CAD build for the part. Positions are in the model's coordinates, mm. Give positions to 0.01 mm unless a question says otherwise; leave off trailing zeros. Write each loop counter-clockwise with the first axis right and the second up, starting at its lowest first coordinate (ties: lowest second). Pieces come first, ordered by that corner, then holes. Notation, with made-up numbers: (71, -38) - (77, -38) arc R13 cw to (77, -20) - close; hole circle Ø4 at (-21, 33.5). An arc over 180 degrees is marked (long way). Answer as a JSON object with one key per item and string values.
from build123d import *

# Parameters (mm, degrees)
SKETCH2_R           = 5.08
BOSS_EXTRUDE1_DEPTH = 6.35
FILLET1_R           = 6.35
FILLET2_R           = 6.35


with BuildPart() as part:
    # Sketch2 → Boss-Extrude1 (new body)
    with BuildSketch(Plane(origin=(0, 0, 0), x_dir=(1, 0, 0), z_dir=(0, 1, 0))):
        Polygon((-152.4, 152.4), (-152.4, -152.4), (152.4, -152.4), (152.4, 142.494), (152.4, 152.4), (142.494, 152.4), align=None)
        with Locations((-139.7, -139.7)):
            Circle(SKETCH2_R, mode=Mode.SUBTRACT)
        with Locations((-56.896, -76.2)):
            Circle(SKETCH2_R, mode=Mode.SUBTRACT)
        with Locations((139.7, -139.7)):
            Circle(SKETCH2_R, mode=Mode.SUBTRACT)
        with Locations((56.896, -76.2)):
            Circle(SKETCH2_R, mode=Mode.SUBTRACT)
        with Locations((-139.7, 139.7)):
            Circle(SKETCH2_R, mode=Mode.SUBTRACT)
        with Locations((-31.496, 88.9)):
            Circle(SKETCH2_R, mode=Mode.SUBTRACT)
        with Locations((31.496, 88.9)):
            Circle(SKETCH2_R, mode=Mode.SUBTRACT)
        with Locations((139.7, 139.7)):
            Circle(SKETCH2_R, mode=Mode.SUBTRACT)
    extrude(amount=BOSS_EXTRUDE1_DEPTH)

    # Fillet1
    fillet1_edges = [part.edges().sort_by_distance(p)[0] for p in [
        (-152.4, 3.175, 152.4),
    ]]
    fillet(fillet1_edges, radius=FILLET1_R)

    # Fillet2
    fillet2_edges = [part.edges().sort_by_distance(p)[0] for p in [
        (-152.4, 3.175, -152.4),
        (152.4, 3.175, -152.4),
        (152.4, 3.175, 152.4),
    ]]
    fillet(fillet2_edges, radius=FILLET2_R)


solid = part.part
(1) Flat gauge pins, fed straight in: P1, Ø16.5, axis at x = 139.7, z = 139.7, coming from the -Y side; P2, Ø6, axis at x = 56.896, z = 76.2, coming from the +Y side. Where does each tip first touch, or does it go through?
Answer key:
{"P1": "stops at y = 0", "P2": "passes through"}
(2) Saw through at B-B, the plane z = -88.9. Give the cut face in (x, y).
Answer key:
{"outline": "(-152.4, 0) - (-36.58, 0) - (-36.58, 6.35) - (-152.4, 6.35) - close; (-26.42, 0) - (26.42, 0) - (26.42, 6.35) - (-26.42, 6.35) - close; (36.58, 0) - (152.4, 0) - (152.4, 6.35) - (36.58, 6.35) - close"}
(3) Probe L1, parallel to Z at x = 139.7, y = 5; L2, parallel to X at y = 3, z = -88.9. List the from-to ranges inside material, lowest first. Write a range as [from, to].
Answer key:
{"L1": "z = [-152.4, -144.78], [-134.62, 134.62], [144.78, 152.4]", "L2": "x = [-152.4, -36.58], [-26.42, 26.42], [36.58, 152.4]"}
(4) Pull direction Z, two halves, no side cores. Call faces 1 (the face through (-58, 3.13, 81.16)), 2 (the face through (-2, 0, -2)): pulls with the +Z half, pulls with the -Z half, needs draft (parallel to the pull), parting line crosses it, or undercut.
Answer key:
{"face 1": "undercut", "face 2": "needs draft"}
(5) Saw through at A-A, the plane x = -139.7. Give the cut face in (y, z), and give its area (3 significant figures).
Answer key:
{"outline": "(0, -152.4) - (6.35, -152.4) - (6.35, -144.78) - (0, -144.78) - close; (0, -134.62) - (6.35, -134.62) - (6.35, 134.62) - (0, 134.62) - close; (0, 144.78) - (6.35, 144.78) - (6.35, 152.4) - (0, 152.4) - close", "area": "1,810 mm²"}
